from build123d import *

# Parameters (mm, degrees)
F0_R     = 21.2328125
F1_DEPTH = 12.7
F2_DEPTH = 385


# Not quite as in the source:
# - an extrude ends at something that could not be found from the text; its depth is read off the source's solid


with BuildPart() as f1:
    # F0 (on Front) → F1 (new body)
    with BuildSketch(Plane.XZ):
        Polygon((177.8, 17.1069), (177.8, 63.5), (131.4069, 63.5), (-131.4069, 63.5), (-177.8, 63.5), (-177.8, 17.1069), (-177.8, -63.5), (177.8, -63.5), align=None)
        with Locations((-131.4069, 17.1069)):
            Circle(F0_R, mode=Mode.SUBTRACT)
        with Locations((131.4069, 17.1069)):
            Circle(F0_R, mode=Mode.SUBTRACT)
    extrude(amount=F1_DEPTH)

    # F0 (on Front) → F2 (cut, through all)
    with BuildSketch(Plane.XZ):
        Polygon((177.8, 17.1069), (177.8, 63.5), (131.4069, 63.5), (-131.4069, 63.5), (-177.8, 63.5), (-177.8, 17.1069), (-177.8, -63.5), (177.8, -63.5), align=None)
        with Locations((-131.4069, 17.1069)):
            Circle(F0_R, mode=Mode.SUBTRACT)
        with Locations((131.4069, 17.1069)):
            Circle(F0_R, mode=Mode.SUBTRACT)
    extrude(amount=-F2_DEPTH, mode=Mode.SUBTRACT)


solid = f1.part
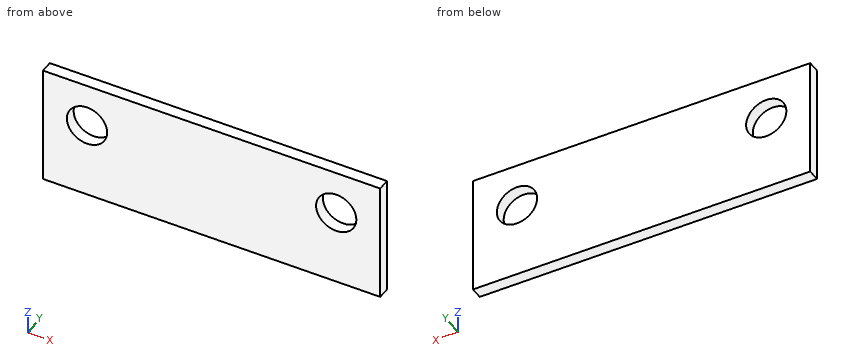
The model under review builds one solid part; all positions refer to its coordinate system, in mm. Coordinates: 2 decimals unless noted, no trailing zeros. Loops run counter-clockwise (first coordinate to the right, second up) from the corner with the lowest first, then second, coordinate; pieces in that order, holes last. Notation, with made-up numbers: (14.25, 53) -> (18.25, 53) arc R16 ccw to (18.25, 60) -> close; hole circle Ø7 at (61, 25). An arc over 180 degrees is marked (long way). Use a Markdown table: item, result. Add a question column.
1. Add section A-A on x = 130. Write out the cut boundary in (y, z).
2. To check wall thickness, follow line 1 (X direction, y = -3.25, z = 22); line 2 (X direction, y = -11, z = 34); line 3 (Z direction, x = 129.5, y = -6.75). State the ranges of each line that lie inside material, in increasing order.
3. Add section B-B on z = 5. Write out the cut boundary in (x, y).
4. Add section D-D on x = -143.5. Write out the cut boundary in (y, z), plus the area to 3 significant figures.
5. Add section C-C on y = -10.5. Write out the cut boundary in (x, z), plus the area to 3 significant figures.
Returned:
| question | item | result |
|---|---|---|
| 1 | outline | (-12.7, -63.5) -> (0, -63.5) -> (0, -4.08) -> (-12.7, -4.08) -> close; (-12.7, 38.29) -> (0, 38.29) -> (0, 63.5) -> (-12.7, 63.5) -> close |
| 2 | line 1 | x = -177.8 to -152.07, -110.75 to 110.75, 152.07 to 177.8 |
| 2 | line 2 | x = -177.8 to -144.27, -118.54 to 118.54, 144.27 to 177.8 |
| 2 | line 3 | z = -63.5 to -4.04, 38.25 to 63.5 |
| 3 | outline | (-177.8, -12.7) -> (-148.85, -12.7) -> (-148.85, 0) -> (-177.8, 0) -> close; (-113.96, -12.7) -> (113.96, -12.7) -> (113.96, 0) -> (-113.96, 0) -> close; (148.85, -12.7) -> (177.8, -12.7) -> (177.8, 0) -> (148.85, 0) -> close |
| 4 | outline | (-12.7, -63.5) -> (0, -63.5) -> (0, -0.35) -> (-12.7, -0.35) -> close; (-12.7, 34.56) -> (0, 34.56) -> (0, 63.5) -> (-12.7, 63.5) -> close |
| 4 | area | 1,170 mm² |
| 5 | outline | (-177.8, -63.5) -> (177.8, -63.5) -> (177.8, 63.5) -> (-177.8, 63.5) -> close; hole circle Ø42.47 at (-131.41, 17.11); hole circle Ø42.47 at (131.41, 17.11) |
| 5 | area | 42,300 mm² |
